For this review, use the dimensioned drawing (mm, ordinates from the lowest corner) and the shaded views. Round coordinates to 2 decimals unless told otherwise and drop trailing zeros. Loops run counter-clockwise (first coordinate to the right, second up) from the corner with the lowest first, then second, coordinate; pieces in that order, holes last. Notation, with made-up numbers: M -20,86 L -5,86 A24 ccw -5,111 Z; hole C -2.5,61 d2. An arc over 180 degrees is marked long. One line per item, written item: value. Start each with the question number.
Item 1: We need section A-A (y = 158.5). Write out the cut boundary in (x, z).
Item 2: For line 1 along Y through (x, z) = (98.5, 3.05); line 2 along Z through (x, y) = (39.5, 83), list the stretches that pass through material, from the lowest coordinate up.
Item 3: We need section B-B (x = 98.5). Write out the cut boundary in (y, z), then the cut area to 4 significant figures.
Item 4: Mouldability with a two-part tool opening along X and no side actions: class the marked faces 1, 2 and 3 as released by +X, released by -X, zero draft, split by the parting line, or undercut.
Item 5: Clearance check with a flat-ended pin moving along its axis: pin 1 (10 mm diameter, centred on x = 127, y = 57, fed in from -Z). State where the tip first meets the part, or that it passes through.
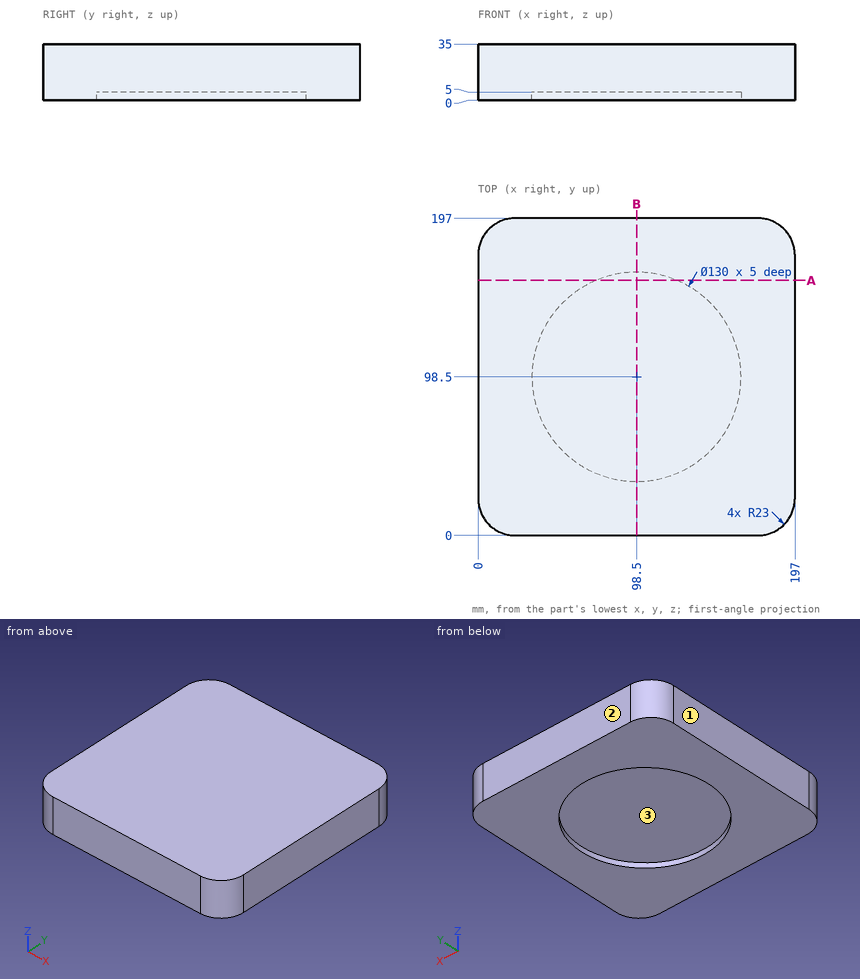
A:
1. outline: M 0,0 L 73.5,0 L 73.5,5 L 123.5,5 L 123.5,0 L 197,0 L 197,35 L 0,35 Z
2. line 1: 0 to 33.5, 163.5 to 197
2. line 2: 5 to 35
3. outline: M 0,0 L 33.5,0 L 33.5,5 L 163.5,5 L 163.5,0 L 197,0 L 197,35 L 0,35 Z
3. area: 6,245 mm2
4. face 1: released by -X
4. face 2: zero draft
4. face 3: undercut
5. pin 1: z = 5
